Check sheet for the modelled part. Datum: model origin and axes. Units: mm. A direction names the side the tool comes from. Give positions to 0.01 mm unless a question says otherwise; leave off trailing zeros. Order: outer loops, then holes, each group sorted by start corner. A loop starts at its lowest first (then second) coordinate and runs counter-clockwise, first axis right, second up.
```python
from build123d import *

# Parameters (mm, degrees)
F0_R     = 7.5
F1_DEPTH = 1.75
F2_R     = 8.5
F2_R_2   = 7.5
F3_DEPTH = 2.75
F4_R     = 10
F4_R_2   = 7.5
F5_DEPTH = 1.5


with BuildPart() as f1:
    # F0 (on Front) → F1 (new body, symmetric)
    with BuildSketch(Plane.XZ):
        with BuildLine():
            Line((-13.891386, 16.048208), (-29.641638, 0))
            ThreePointArc((-29.641638, 0), (-29.452592, -5.025263), (-25.179131, -7.676025))
            add(Edge.make_bspline(
                [(-25.179131, -7.676025), (-18.558836, -7.633325), (-17.581457, -10.063985), (-16.679482, -11.024288)],
                knots=[0, 0, 0, 0, 9.135366, 9.135366, 9.135366, 9.135366], degree=3))
            ThreePointArc((-16.679482, -11.024288), (-11.621852, -14.676658), (-5.63849, -16.44267))
            Line((-5.63849, -16.44267), (4.816984, -16.44267))
            ThreePointArc((4.816984, -16.44267), (11.240893, -14.812063), (16.679482, -11.024288))
            add(Edge.make_bspline(
                [(25.179131, -7.676025), (18.558836, -7.633325), (17.581457, -10.063985), (16.679482, -11.024288)],
                knots=[0, 0, 0, 0, 9.135366, 9.135366, 9.135366, 9.135366], degree=3))
            ThreePointArc((25.179131, -7.676025), (29.452592, -5.025263), (29.641638, 0))
            Line((29.641638, 0), (13.891386, 16.048208))
            ThreePointArc((13.891386, 16.048208), (12.113511, 17.071286), (10.087852, 17.394136))
            Line((10.087852, 17.394136), (-9.978892, 17.39047))
            ThreePointArc((-9.978892, 17.39047), (-12.062035, 17.089223), (-13.891386, 16.048208))
        make_face()
        with Locations((0, -1.673267)):
            Circle(F0_R, mode=Mode.SUBTRACT)
        with BuildLine():
            Line((-8.652875, 11.747209), (-25.002061, -4.602077))
            ThreePointArc((-25.002061, -4.602077), (-25.997431, -5.014338), (-26.992801, -4.602077))
            Line((-26.992801, -4.602077), (-27.823672, -3.771305))
            ThreePointArc((-27.823672, -3.771305), (-28.235982, -2.775914), (-27.823572, -1.780565))
            Line((-27.823572, -1.780565), (-11.474387, 14.56872))
            ThreePointArc((-11.474387, 14.56872), (-10.479017, 14.980981), (-9.483647, 14.56872))
            Line((-9.483647, 14.56872), (-8.652775, 13.737948))
            ThreePointArc((-8.652775, 13.737948), (-8.240465, 12.742558), (-8.652875, 11.747209))
        make_face(mode=Mode.SUBTRACT)
        with BuildLine():
            ThreePointArc((9.483647, 14.56872), (10.479017, 14.980981), (11.474387, 14.56872))
            Line((11.474387, 14.56872), (27.823572, -1.780565))
            ThreePointArc((27.823572, -1.780565), (28.235982, -2.775914), (27.823672, -3.771305))
            Line((27.823672, -3.771305), (26.992801, -4.602077))
            ThreePointArc((26.992801, -4.602077), (25.997431, -5.014338), (25.002061, -4.602077))
            Line((25.002061, -4.602077), (8.652875, 11.747209))
            ThreePointArc((8.652875, 11.747209), (8.240465, 12.742558), (8.652775, 13.737948))
            Line((8.652775, 13.737948), (9.483647, 14.56872))
        make_face(mode=Mode.SUBTRACT)
    extrude(amount=F1_DEPTH, both=True)

    # F2 (on Front) → F3 (join, symmetric)
    with BuildSketch(Plane.XZ):
        with Locations((0, -1.673267)):
            Circle(F2_R)
        with Locations((0, -1.673267)):
            Circle(F2_R_2, mode=Mode.SUBTRACT)
    extrude(amount=F3_DEPTH, both=True)

    # F4 (on face) → F5 (join)
    with BuildSketch(Plane.XZ.offset(2.75)):
        with Locations((0, -1.673267)):
            Circle(F4_R)
        with Locations((0, -1.673267)):
            Circle(F4_R_2, mode=Mode.SUBTRACT)
    extrude(amount=F5_DEPTH)


solid = f1.part
```
(1) Cross-section at B-B on z = 1. Enter the section's corners in (x, y).
Response values:
outline: (-28.66, -1.75) - (-25.04, -1.75) - (-25.04, 1.75) - (-28.66, 1.75) - close; (-19.4, -1.75) - (-8.07, -1.75) - (-8.07, -2.75) - (-9.64, -2.75) - (-9.64, -4.25) - (-7.01, -4.25) - (-7.01, 2.75) - (-8.07, 2.75) - (-8.07, 1.75) - (-19.4, 1.75) - close; (7.01, -4.25) - (9.64, -4.25) - (9.64, -2.75) - (8.07, -2.75) - (8.07, -1.75) - (19.4, -1.75) - (19.4, 1.75) - (8.07, 1.75) - (8.07, 2.75) - (7.01, 2.75) - close; (25.04, -1.75) - (28.66, -1.75) - (28.66, 1.75) - (25.04, 1.75) - close
(2) Cross-section at D-D on x = 0. Enter the section's corners in (y, z), then the cut area to 3 significant figures.
Response values:
outline: (-4.25, -11.67) - (-2.75, -11.67) - (-2.75, -10.17) - (-1.75, -10.17) - (-1.75, -16.44) - (1.75, -16.44) - (1.75, -10.17) - (2.75, -10.17) - (2.75, -9.17) - (-4.25, -9.17) - close; (-4.25, 5.83) - (2.75, 5.83) - (2.75, 6.83) - (1.75, 6.83) - (1.75, 17.39) - (-1.75, 17.39) - (-1.75, 6.83) - (-2.75, 6.83) - (-2.75, 8.33) - (-4.25, 8.33) - close
area: 77.4 mm2
(3) Gauge pin test, flat ends, axial feed: pin 1 Ø5 at (x, z) = (-12.5, 8) entering from -Y; pin 2 Ø6 at (x, z) = (17.5, 7.5) entering from +Y; pin 3 Ø2 at (x, y) = (13.5, 1) entering from +Z. Record the tip position at first contact, or that the pin passes through.
Response values:
pin 1: stops at y = -1.75
pin 2: stops at y = 1.75
pin 3: stops at z = 16.92
(4) Material ranges on L1, parallel to Z at x = 0, y = 1.25; L2, parallel to X at y = 0.25, z = 1; L3, parallel to Y at x = 8, z = 2, recorded low to high.
Response values:
L1: z = -16.44 to -9.17, 5.83 to 17.39
L2: x = -28.66 to -25.04, -19.4 to -7.01, 7.01 to 19.4, 25.04 to 28.66
L3: y = -4.25 to -2.75, -1.75 to 1.75
(5) Cross-section at A-A on x = 15.5. Enter the section's corners in (y, z), then the cut area to 3 significant figures.
Response values:
outline: (-1.75, -12.11) - (1.75, -12.11) - (1.75, 4.9) - (-1.75, 4.9) - close; (-1.75, 10.54) - (1.75, 10.54) - (1.75, 14.41) - (-1.75, 14.41) - close
area: 73.1 mm2
(6) Release check for a two-part mould opening along Z. For faces 1 (the face through (16.9, 0, 3.5)), 2 (the face through (-6.745, 2.243, -6.845)), 3 (the face through (-7, 1.75, 4)) record: released by +Z, released by -Z, zero draft, split by the parting line, or undercut.
Response values:
face 1: undercut
face 2: split by the parting line
face 3: zero draft
(7) Set-up check for faces 4 (the face through (-16.7, 0, 3.7)), 5 (the face through (-7, -1.75, 4)), 6 (the face through (29.415, -0.024, -5.088)): record each of +Z, -Z, +X, -X, +Y, -Y from which the full face is reachable in a straight line by a thin tool's end or side.
Response values:
face 4: +Y, -Y
face 5: none
face 6: +X, +Y, -Y
(8) Cross-section at C-C on z = -7. Enter the section's corners in (x, y).
Response values:
outline: (-27.45, -1.75) - (-6.62, -1.75) - (-6.62, -2.75) - (-8.46, -2.75) - (-8.46, -4.25) - (-5.28, -4.25) - (-5.28, 2.75) - (-6.62, 2.75) - (-6.62, 1.75) - (-27.45, 1.75) - close; (5.28, -4.25) - (8.46, -4.25) - (8.46, -2.75) - (6.62, -2.75) - (6.62, -1.75) - (27.45, -1.75) - (27.45, 1.75) - (6.62, 1.75) - (6.62, 2.75) - (5.28, 2.75) - close
